Autodesk Inventor part; units mm, degrees
ref_plane "YZ Plane" through (0, 0, 0) normal (1, 0, 0) x (0, 1, 0)
ref_plane "XZ Plane" through (0, 0, 0) normal (0, 1, 0) x (-1, 0, 0)
ref_plane "XY Plane" through (0, 0, 0) normal (0, 0, 1) x (1, 0, 0)
sketch "Sketch1" plane through (0, 0, 0) normal (0, 0, 1) x (1, 0, 0)
  line L0 (-25, -10) -> (25, -10)
  line L1 (25, -10) -> (25, 10)
  line L2 (25, 10) -> (-25, 10)
  line L3 (-25, 10) -> (-25, -10)
  line L4 (-25, -10) -> (25, 10) construction
  line L5 (25, -10) -> (-25, 10) construction
  circle A0 centre (-7.427, -0.0759) radius 3.5
  circle A1 centre (8.8633, -0.0759) radius 3.5
  line L6 (0.033, 2.0872) -> (2.5566, 2.0872)
  line L7 (2.5566, 2.0872) -> (2.5566, 1.2559)
  line L8 (2.5566, 1.2559) -> (0.033, 1.2559)
  line L9 (0.033, 1.2559) -> (0.033, 2.0872)
  line L10 (0.033, 2.0872) -> (2.5566, 1.2559) construction
  line L11 (2.5566, 2.0872) -> (0.033, 1.2559) construction
  circle A2 centre (-7.427, -0.0759) radius 2.5
  circle A3 centre (8.8633, -0.0759) radius 2.5
  point P0 (0, 0)
  point P1 (1.2948, 1.6716)
  dimension "d0" = 7
  dimension "d1" = 7
  dimension "d11" = 5
  dimension "d12" = 5
  dimension "d28" = 50
  dimension "d29" = 20
extrude "Extrusion1" add sketch "Sketch1" against normal blind 10 contours L3 L2 L1 L0 | A0 | A1 | L6 L7 L8 L9 | A2 | A3
extrude "Extrusion2" add sketch "Sketch1" along normal blind 1.5 contours A0 | A2
extrude "Extrusion3" add sketch "Sketch1" along normal blind 2 contours A1 | A3
extrude "Extrusion4" add sketch "Sketch1" along normal blind 0.5 contours L6 L7 L8 L9
fillet "Fillet1" radius 0.1 4 edges at (1.2948, 2.0872, 0.5) (2.5566, 1.6716, 0.5) (1.2948, 1.2559, 0.5) (0.033, 1.6716, 0.5)
extrude "Extrusion5" add sketch "Sketch1" along normal blind 5 contours A2
extrude "Extrusion6" add sketch "Sketch1" along normal blind 5 contours A3
sketch "Sketch3" plane through (-25, 10, 0) normal (0, 1, 0) x (1, 0, 0)
  circle A0 centre (29.4869, 3.1475) radius 0.75
  circle A1 centre (27.0793, 3.1475) radius 0.75
  circle A2 centre (25, 3.1475) radius 0.75
  circle A3 centre (22.4188, 3.1475) radius 0.75
  point P0 (25, 0)
  dimension "d19" = 1.5
  dimension "d20" = 1.5
  dimension "d21" = 1.5
  dimension "d22" = 1.5
extrude "Extrusion8" add sketch "Sketch3" along normal blind 10 contours A0 | A2 | A3
extrude "Extrusion9" add sketch "Sketch3" along normal blind 10 contours A1
sketch "Sketch4" plane through (0, 0, 0) normal (0, 0, 1) x (1, 0, 0)
  point P0 (0, 0)
properties part number "ultrasonic sensor"
Can you work these out from the model? Positions are in its coordinate system, mm. A direction names the side the tool comes from. Coordinates: 2 decimals unless noted, no trailing zeros. Write each loop counter-clockwise with the first axis right and the second up, starting at its lowest first coordinate (ties: lowest second). Pieces come first, ordered by that corner, then holes. Notation, with made-up numbers: (38, 82.25) -> (54, 82.25) arc R20 cw to (54, 91.25) -> close; hole circle Ø2 at (43, 38). An arc over 180 degrees is marked (long way). Write each question's results on one line, items separated by ' | '. Start each with the question number.
Q1. Imagine slicing it at B-B (z = -5.75). Write out the boundary of the cut face in (x, y).
Q2. If I drill on probe 1 along Z at (x, y) = (-11.5, -1.5); probe 2 along Y at (x, z) = (-13, -3.25); probe 3 along Y at (x, z) = (9, 1.75), over which ranges is the centre line in solid material (lowest first)?
Q3. Imagine slicing it at C-C (y = 6.5). Write out the boundary of the cut face in (x, z).
Q4. Imagine slicing it at D-D (z = 3). Write out the boundary of the cut face in (x, y), then the cut area to 3 significant figures.
Q5. On a 3-axis mill with a long thin cutter (end or side, diameter ignored), from which of +Z, -Z, +X, -X, +Y, -Y can I reach the whole of each face in a straight line? I mean faces 4 (the face through (0, 20, -3)), 5 (the face through (-8.19, 3.34, 0.74)), 6 (the face through (-0.16, 14.93, -3.88)). Say none if no direction works.
Q6. We'd pull the mould along X, two halves only. Please class faces 1 (the face through (6, 1, 2)), 2 (the face through (-25, 0, -5)), 3 (the face through (9, 0, 5)): +X half, -X half, draft (parallel to the pull), parting line (faces both ways), or undercut.
Q7. I'm going to push flat-ended pins straight in: pin 1 (4 mm diameter, centred on x = -17, z = -6, fed in from +Y); pin 2 (1 mm diameter, centred on y = 0.5, z = 3, fed in from -X); pin 3 (1.5 mm diameter, centred on x = -18.5, y = -4.5, fed in from +Z). Where does each tip first touch, or does it pass through?
Q8. Imagine slicing it at A-A (x = 9.5). Write out the boundary of the cut face in (y, z).
Taken from the geometry:
1) outline: (-25, -10) -> (25, -10) -> (25, 10) -> (-25, 10) -> close
2) probe 1: z = -10 to 0 | probe 2: y = -10 to 10 | probe 3: y = -3.57 to 3.42
3) outline: (-25, -10) -> (25, -10) -> (25, 0) -> (-25, 0) -> close
4) outline: circle Ø5 at (-7.43, -0.08); circle Ø5 at (8.86, -0.08) | area: 39.3 mm^2
5) face 4: +Z, -Z, +X, -X, +Y | face 5: +Z | face 6: +Y
6) face 1: undercut | face 2: -X half | face 3: draft
7) pin 1: stops at y = 10 | pin 2: stops at x = -9.93 | pin 3: stops at z = 0
8) outline: (-10, -10) -> (10, -10) -> (10, 0) -> (3.37, 0) -> (3.37, 2) -> (2.34, 2) -> (2.34, 5) -> (-2.49, 5) -> (-2.49, 2) -> (-3.52, 2) -> (-3.52, 0) -> (-10, 0) -> close
